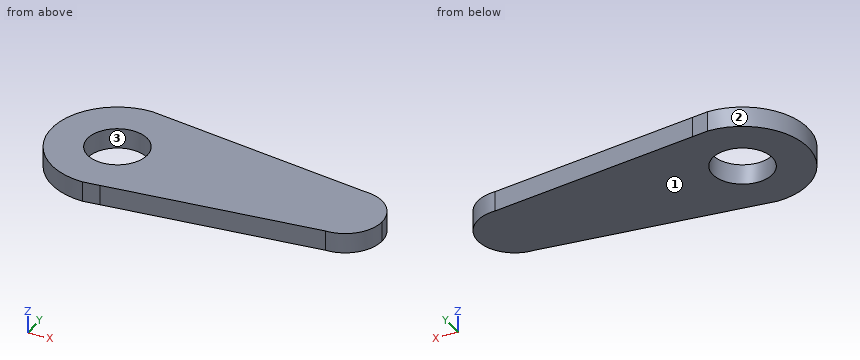
from build123d import *

# Parameters (mm, degrees)
F0_R     = 2.9612883312
F1_DEPTH = 2
F2_R     = 0.988841467
F3_DEPTH = 10


with BuildPart() as f1:
    # F0 (on Top) → F1 (new body)
    with BuildSketch(Plane.XY):
        with BuildLine():
            Line((1.6245851515, 6.3095047445), (0, 6.5152994586))
            ThreePointArc((0, 6.5152994586), (-6.5152994586, 0), (0, -6.5152994586))
            Line((0, -6.5152994586), (1.6245851515, -6.3095047445))
            ThreePointArc((1.6245851515, -6.3095047445), (5.1494555923, -3.9915202792), (6.5152994586, 0))
            ThreePointArc((6.5152994586, 0), (5.1494555923, 3.9915202792), (1.6245851515, 6.3095047445))
        make_face()
        Circle(F0_R, mode=Mode.SUBTRACT)
        with BuildLine():
            Line((22.574134171, 3.6557155928), (1.6245851515, 6.3095047445))
            ThreePointArc((1.6245851515, 6.3095047445), (5.1494555923, 3.9915202792), (6.5152994586, 0))
            ThreePointArc((6.5152994586, 0), (5.1494555923, -3.9915202792), (1.6245851515, -6.3095047445))
            Line((1.6245851515, -6.3095047445), (22.574134171, -3.6557155928))
            ThreePointArc((22.574134171, -3.6557155928), (18.9184185782, 0), (22.574134171, 3.6557155928))
        make_face()
        with BuildLine():
            ThreePointArc((26.2298497639, 0), (25.1591154568, 2.5849812858), (22.574134171, 3.6557155928))
            ThreePointArc((22.574134171, 3.6557155928), (18.9184185782, 0), (22.574134171, -3.6557155928))
            ThreePointArc((22.574134171, -3.6557155928), (25.1591154568, -2.5849812858), (26.2298497639, 0))
        make_face()
    extrude(amount=F1_DEPTH)

    # F2 (on face) → F3 (cut)
    with BuildSketch(Plane.XY.offset(2)):
        with Locations((22.574134171, 0)):
            Circle(F2_R)
    extrude(amount=F3_DEPTH, mode=Mode.SUBTRACT)


solid = f1.part
Read the model definition and answer for the solid it produces. Units are mm, in the model's axes. Face numbers are marked on the shaded views. Give positions to 0.01 mm unless a question says otherwise; leave off trailing zeros. Write each loop counter-clockwise with the first axis right and the second up, starting at its lowest first coordinate (ties: lowest second). Pieces come first, ordered by that corner, then holes. Notation, with made-up numbers: M 68.25,3 L 107.25,3 A20 cw 107.25,14 Z; hole C 13,12 d4. An arc over 180 degrees is marked long. One line per item, written item: value. Start each with the question number.
(1) Find section B-B (y = 2). Determine the outline of the cut face in (x, z).
(2) Find the intervals of material crossed by line 1 (Y direction, x = 0, z = 1.05); line 2 (X direction, y = 0.5, z = 0.9); line 3 (Y direction, x = 1, z = 1.2), in increasing order.
(3) A flat-ended cylindrical pin translates along its axis: pin 1 Ø5.5 at (x, y) = (0, 0) entering from -Z. Find the tip coordinate at first contact, or state that the pin passes through.
(4) Determine the mould class of the marked faces 1, 2 and 3 for opening direction Y: pulls with the +Y half, pulls with the -Y half, needs draft (parallel to the pull), parting line crosses it, or undercut.
(5) Find section A-A (z = 0.5). Determine the outline of the cut face in (x, y).
(6) Find section C-C (x = 19.5). Determine the outline of the cut face in (y, z), plus the area to 3 significant figures.
(7) Find section D-D (y = -4.25). Determine the outline of the cut face in (x, z).
Results below:
1. outline: M -6.2,0 L -2.18,0 L -2.18,2 L -6.2,2 Z; M 2.18,0 L 25.63,0 L 25.63,2 L 2.18,2 Z
2. line 1: y = -6.52 to -2.96, 2.96 to 6.52
2. line 2: x = -6.5 to -2.92, 2.92 to 26.2
2. line 3: y = -6.39 to -2.79, 2.79 to 6.39
3. pin 1: passes through
4. face 1: needs draft
4. face 2: parting line crosses it
4. face 3: undercut
5. outline: M 0,-6.52 L 22.57,-3.66 A3.66 ccw 22.57,3.66 L 0,6.52 A6.52 ccw Z; hole C 0,0 d5.92
6. outline: M -4.05,0 L 4.05,0 L 4.05,2 L -4.05,2 Z
6. area: 16.2 mm^2
7. outline: M -4.94,0 L 17.88,0 L 17.88,2 L -4.94,2 Z
